```python
from build123d import *

# Parameters (mm, degrees)
F1_DEPTH = 3
F2_DEPTH = 75
F3_DEPTH = 15
F4_SIZE  = 7
F5_W     = 42
F5_H     = 3
F6_DEPTH = 60
F8_DEPTH = 15


with BuildPart() as f1:
    # F0 (on Top) → F1 (new body)
    with BuildSketch(Plane.XY):
        Polygon((0, 60), (-12.5, 60), (-12.5, -21), (45, -21), (45, 0), (0, 0), align=None)
    extrude(amount=F1_DEPTH)

    # F0 (on Top) → F2 (join)
    with BuildSketch(Plane.XY):
        Polygon((-12.5, -21), (-12.5, 60), (-15.5, 60), (-15.5, -24), (45, -24), (45, -21), align=None)
    extrude(amount=F2_DEPTH)

    # F0 (on Top) → F3 (join)
    with BuildSketch(Plane.XY):
        Polygon((3, 60), (0, 60), (0, 0), (45, 0), (45, 3), (3, 3), align=None)
    extrude(amount=F3_DEPTH)

    # F4
    f4_edges = [f1.edges().sort_by_distance(p)[0] for p in [
        (-12.5, -21, 39),
    ]]
    chamfer(f4_edges, length=F4_SIZE)

    # F5 (on face) → F6 (join, through all)
    with BuildSketch(Plane.XY.offset(15)):
        with Locations((24, 1.5)):
            Rectangle(F5_W, F5_H)
    extrude(amount=F6_DEPTH)

    # F7 (on face) → F8 (join, through all)
    with BuildSketch(Plane(origin=(0, 0, 0), x_dir=(1, 0, 0), z_dir=(0, 0, -1))):
        Polygon((3, -45), (45, -3), (3, -3), align=None)
    extrude(amount=-F8_DEPTH)


solid = f1.part
```
Input: part model. Units: mm. Frame: model coordinates. A direction names the side the tool comes from. Give positions to 0.01 mm unless a question says otherwise; leave off trailing zeros. Order: outer loops, then holes, each group sorted by start corner. A loop starts at its lowest first (then second) coordinate and runs counter-clockwise, first axis right, second up. Notation, with made-up numbers: M 19,82.5 L 36,82.5 A13 ccw 36,89.5 Z; hole C 52,88 d1. An arc over 180 degrees is marked long. One line per question, with ' | ' between items. Start each with the question number.
1. First-contact query: pin 1 Ø5 at (x, z) = (-4.5, 24) entering from +Y; pin 2 Ø5 at (y, z) = (22, 41.5) entering from +X; pin 3 Ø25 at (x, z) = (28.5, 46) entering from +Y; pin 4 Ø10 at (x, y) = (10, -5.5) entering from -Z. Flat tips, straight axial feed; report the tip coordinate or a pass-through.
2. Section query B-B (y = 35.5). Return the cut outline in (x, z), and give its area (3 significant figures).
3. Section query C-C (x = 18). Return the cut outline in (y, z), and give its area (3 significant figures).
4. Section query A-A (z = 10). Return the cut outline in (x, y).
5. Access query for faces 1 (the face through (22, 0, 38)), 2 (the face through (-9, -17.5, 38.5)), 3 (the face through (0, 30, 9)). Directions: +Z, -Z, +X, -X, +Y, -Y. A direction counts if a zero-diameter tool reaches every point of the face in a straight line with its end or side. Return the directions, or none.
6. Section query D-D (z = 36). Return the cut outline in (x, y), and give its area (3 significant figures).
7. Material intervals for probe 1 along Y at (x, z) = (30.5, 68); probe 2 along Z at (x, y) = (-3.5, 4); probe 3 along X at (y, z) = (-6.5, 17), sorted ascending. Write a range as [from, to].
Here are the results:
1) pin 1: y = -19.5 | pin 2: x = -12.5 | pin 3: y = 3 | pin 4: z = 0
2) outline: M -15.5,0 L 12.5,0 L 12.5,15 L 0,15 L 0,3 L -12.5,3 L -12.5,75 L -15.5,75 Z | area: 450 mm²
3) outline: M -24,0 L 30,0 L 30,15 L 3,15 L 3,75 L 0,75 L 0,3 L -21,3 L -21,75 L -24,75 Z | area: 918 mm²
4) outline: M -15.5,-24 L 45,-24 L 45,-21 L -5.5,-21 L -12.5,-14 L -12.5,60 L -15.5,60 Z; M 0,0 L 45,0 L 45,3 L 3,45 L 3,60 L 0,60 Z
5) face 1: +Z, +X | face 2: +Z, +X, +Y | face 3: +Z, +Y
6) outline: M -15.5,-24 L 45,-24 L 45,-21 L -5.5,-21 L -12.5,-14 L -12.5,60 L -15.5,60 Z; M 3,0 L 45,0 L 45,3 L 3,3 Z | area: 575 mm²
7) probe 1: [-24, -21], [0, 3] | probe 2: [0, 3] | probe 3: [-15.5, -12.5]
